Part model, mm, in its own coordinate system. Coordinates: 2 decimals unless noted, no trailing zeros. Loops run counter-clockwise (first coordinate to the right, second up) from the corner with the lowest first, then second, coordinate; pieces in that order, holes last. Notation, with made-up numbers: (3, 32.5) -> (33, 32.5) arc R11 ccw to (33, 42.5) -> close; hole circle Ø8 at (36, -25). An arc over 180 degrees is marked (long way). One line per question, with ' | ' between items. Start each with the question number.
1) Probe L1, parallel to Z at x = 20, y = 15; L2, parallel to X at y = 23, z = 29.5; L3, parallel to Y at x = 52, z = 23.5. List the from-to ranges inside material, lowest first. Write a range as from..to.
2) Cut at C-C (x = 40.5). List the corners of the cut face in (y, z).
3) Cut at A-A (x = 10). List the corners of the cut face in (y, z).
4) Drop flat-ended pins along their axis: pin 1 (13.5 mm diameter, centred on x = -80, z = 26.5, fed in from +Y); pin 2 (6 mm diameter, centred on x = 32.5, y = 19, fed in from +Z); pin 3 (1.5 mm diameter, centred on y = 5.5, z = 38.5, fed in from +X); pin 4 (19 mm diameter, centred on y = 31, z = 17, fed in from -X). Give the stop position or say it passes through.
5) Cut at D-D (y = 29.5). List the corners of the cut face in (x, z).
from build123d import *

# Parameters (mm, degrees)
SALIENTE_EXTRUIR1_DEPTH      = 37.6
SALIENTE_EXTRUIR2_DEPTH      = 5
SALIENTE_EXTRUIR2_DEPTH_BACK = 105
CROQUIS2_R                   = 2
REDONDEO1_R                  = 3
CHAFL_N1_SIZE                = 2
CHAFL_N2_SIZE                = 2
REDONDEO2_R                  = 3
CROQUIS3_R                   = 2.5
SALIENTE_EXTRUIR3_DEPTH      = 5
CROQUIS4_R                   = 1.5
SALIENTE_EXTRUIR4_DEPTH      = 3


with BuildPart() as part:
    # Croquis1 → Saliente-Extruir1 (new body)
    with BuildSketch(Plane.XY):
        Polygon((-62.524392651, 0.371914202), (-62.524392651, -23.628085798), (37.475607349, -23.628085798), (37.475607349, 0.371914202), (67.475607349, 0.371914202), (67.475607349, 22.371914202), (37.475607349, 22.371914202), (37.475607349, 46.371914202), (-62.524392651, 46.371914202), (-62.524392651, 22.371914202), (-92.524392651, 22.371914202), (-92.524392651, 0.371914202), align=None)
    extrude(amount=SALIENTE_EXTRUIR1_DEPTH)

    # Croquis2 → Saliente-Extruir2 (add, two sides: drawn at the far end of the back side and taken through both)
    with BuildSketch(Plane.ZY.offset(62.524392651).offset(-SALIENTE_EXTRUIR2_DEPTH_BACK)):
        with Locations((24, -14.628085798)):
            Circle(CROQUIS2_R)
        with Locations((24, 37.371914202)):
            Circle(CROQUIS2_R)
    extrude(amount=SALIENTE_EXTRUIR2_DEPTH + SALIENTE_EXTRUIR2_DEPTH_BACK)

    # Redondeo1
    redondeo1_edges = [part.edges().sort_by_distance(p)[0] for p in [
        (67.475607349, 22.371914202, 18.8),
        (67.475607349, 0.371914202, 18.8),
    ]]
    fillet(redondeo1_edges, radius=REDONDEO1_R)

    # Chaflán1
    chafl_n1_edges = [part.edges().sort_by_distance(p)[0] for p in [
        (-12.524392651, 46.371914202, 0),
        (-12.524392651, -23.628085798, 0),
    ]]
    chamfer(chafl_n1_edges, length=CHAFL_N1_SIZE)

    # Chaflán2
    chafl_n2_edges = [part.edges().sort_by_distance(p)[0] for p in [
        (-12.524392651, -23.628085798, 37.6),
        (-12.524392651, 46.371914202, 37.6),
    ]]
    chamfer(chafl_n2_edges, length=CHAFL_N2_SIZE)

    # Redondeo2
    redondeo2_edges = [part.edges().sort_by_distance(p)[0] for p in [
        (-92.524392651, 0.371914202, 18.8),
        (-92.524392651, 22.371914202, 18.8),
    ]]
    fillet(redondeo2_edges, radius=REDONDEO2_R)

    # Croquis3 → Saliente-Extruir3 (add)
    with BuildSketch(Plane.XY.offset(37.6)):
        with Locations(Location((-38.524392651, 38.121914202, 0), (0, 0, 180))):
            Circle(CROQUIS3_R)
        with Locations(Location((19.475607349, 38.121914202, 0), (0, 0, 180))):
            Circle(CROQUIS3_R)
        with Locations(Location((-38.524392651, -10.878085798, 0), (0, 0, 180))):
            Circle(CROQUIS3_R)
        with Locations(Location((19.475607349, -10.878085798, 0), (0, 0, 180))):
            Circle(CROQUIS3_R)
    extrude(amount=SALIENTE_EXTRUIR3_DEPTH)

    # Croquis4 → Saliente-Extruir4 (add)
    with BuildSketch(Plane.XY.offset(42.6)):
        with Locations((-38.524392651, 38.121914202)):
            Circle(CROQUIS4_R)
        with Locations((19.475607349, 38.121914202)):
            Circle(CROQUIS4_R)
        with Locations((-38.524392651, -10.878085798)):
            Circle(CROQUIS4_R)
        with Locations((19.475607349, -10.878085798)):
            Circle(CROQUIS4_R)
    extrude(amount=SALIENTE_EXTRUIR4_DEPTH)


solid = part.part
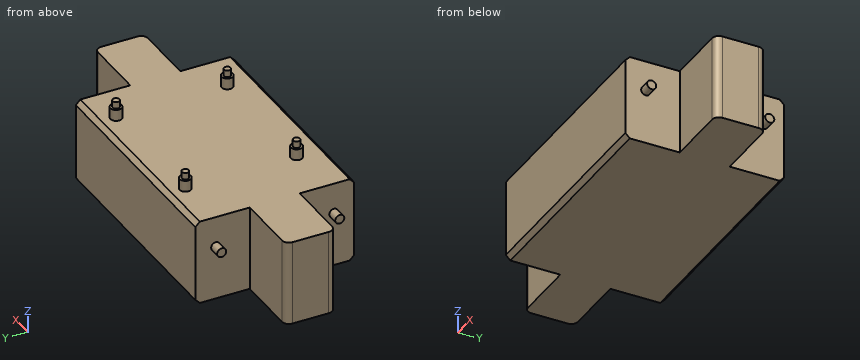
Reported:
1) L1: z = 0..37.6 | L2: x = -62.52..37.48 | L3: y = 0.37..22.37
2) outline: circle Ø4 at (-14.63, 24); (0.37, 0) -> (22.37, 0) -> (22.37, 37.6) -> (0.37, 37.6) -> close; circle Ø4 at (37.37, 24)
3) outline: (-23.63, 2) -> (-21.63, 0) -> (44.37, 0) -> (46.37, 2) -> (46.37, 35.6) -> (44.37, 37.6) -> (-21.63, 37.6) -> (-23.63, 35.6) -> close
4) pin 1: stops at y = 22.37 | pin 2: stops at z = 37.6 | pin 3: passes through | pin 4: stops at x = -91.64
5) outline: (-62.52, 0) -> (37.48, 0) -> (37.48, 37.6) -> (-62.52, 37.6) -> close
